Geometry: final body of the model. Coordinates: model frame, mm. A direction names the side the tool comes from. Coordinates: 2 decimals unless noted, no trailing zeros. Order: outer loops, then holes, each group sorted by start corner. A loop starts at its lowest first (then second) coordinate and runs counter-clockwise, first axis right, second up. Notation, with made-up numbers: M 76.5,40 L 104.5,40 A22 cw 104.5,74 Z; hole C 81,16.25 d11. An arc over 180 degrees is marked long. Write item = value, one per line. Start each with the question number.
Autodesk Inventor part; units mm, degrees
ref_plane "YZ Plane" through (0, 0, 0) normal (1, 0, 0) x (0, 1, 0)
ref_plane "XZ Plane" through (0, 0, 0) normal (0, 1, 0) x (-1, 0, 0)
ref_plane "XY Plane" through (0, 0, 0) normal (0, 0, 1) x (1, 0, 0)
sketch "Sketch1" plane through (0, 0, 0) normal (0, 1, 0) x (-1, 0, 0)
  circle A0 centre (0, 0) radius 40
  circle A1 centre (0, 0) radius 36
  dimension "d1" = 72
  dimension "d8" = 80
extrude "Extrusion1" add sketch "Sketch1" along normal blind 50
sketch "Sketch2" plane through (0, 0, 0) normal (1, 0, 0) x (0, 1, 0)
  line L0 (0, 40) -> (0, -40)
  line L1 (0, -36) -> (19.3804, -30.807)
  line L2 (0, -36) -> (20.8201, -41.5787)
  line L3 (19.3804, -30.807) -> (-2.465, -30.807)
  line L4 (-2.465, -30.807) -> (-2.465, -42.37)
  line L5 (-2.465, -42.37) -> (20.8201, -42.37)
  line L6 (20.8201, -42.37) -> (20.8201, -41.5787)
  line L7 (0, -36) -> (50, -36)
  point P0 (0, 0)
  dimension "d6" = 15
  dimension "d7" = 15
extrude "Extrusion2" cut sketch "Sketch2" along normal mid plane 30
properties part number "Whistle Splitter 40mmR"
Item 1: Section query A-A on z = 0. Output: boundary loops of the cut face in (x, y), and give its area (3 significant figures).
Item 2: Section query B-B on x = 3.5. Output: boundary loops of the cut face in (y, z).
Item 3: Section query C-C on y = 7. Output: boundary loops of the cut face in (x, z).
Item 4: Reachability of faces 4 (the flat face through (15, 5, -34)), 5 (the flat face through (-0.21, 5.701, -37.528)), 6 (the flat face through (6, 0, 36)) from +Z, -Z, +X, -X, +Y, -Y: full face, straight path, thin tool, end or side. Return the list, or none.
Item 5: Draft query along X for faces 1 (the flat face through (33, 50, 15)), 2 (the cylindrical face through (4.686, 24.65, -35.694)), 3 (the cylindrical face through (8.67, 24.65, 39.05)). Return one class per face: pulls with the +X half, pulls with the -X half, needs draft (parallel to the pull), parting line crosses it, or undercut.
Item 6: Material intervals for probe 1 along Z at (x, y) = (0, 19); probe 2 along Z at (x, y) = (0, 11.5), sorted ascending. Write a range as [from, to].
Item 7: Section query D-D on x = -16. Output: boundary loops of the cut face in (y, z).
Item 8: First-contact query: pin 1 (12 mm diameter, centred on y = 39, z = 20, fed in from +X); pin 2 (3 mm diameter, centred on x = 22, y = 33, fed in from -Z); pin 3 (2.5 mm diameter, centred on y = 3, z = -35, fed in from -X); pin 4 (6 mm diameter, centred on x = -27.5, z = -15.5, fed in from -Y). Flat tips, straight axial feed; report the tip coordinate or a pass-through.
Ans:
q1.outline = M -40,0 L -36,0 L -36,50 L -40,50 Z; M 36,0 L 40,0 L 40,50 L 36,50 Z
q1.area = 400 mm^2
q2.outline = M 0,-36 L 14.36,-39.85 L 50,-39.85 L 50,-35.83 L 0.64,-35.83 Z; M 0,35.83 L 50,35.83 L 50,39.85 L 0,39.85 Z
q3.outline = M -12.86,-37.88 L 12.86,-37.88 A40 ccw long Z; hole M -15,-34.12 L -11.47,-34.12 A36 ccw 11.47,-34.12 L 15,-34.12 L 15,-32.73 A36 ccw long -15,-32.73 Z
q4.face_4 = -Y
q4.face_5 = -Z, -Y
q4.face_6 = +Z, -Z, +X, -X, -Y
q5.face_1 = needs draft
q5.face_2 = undercut
q5.face_3 = parting line crosses it
q6.probe_1 = [-40, -36], [36, 40]
q6.probe_2 = [-39.08, -36], [36, 40]
q7.outline = M 0,-36.66 L 50,-36.66 L 50,-32.25 L 0,-32.25 Z; M 0,32.25 L 50,32.25 L 50,36.66 L 0,36.66 Z
q8.pin_1 = 37.47
q8.pin_2 = -34.35
q8.pin_3 = -21.47
q8.pin_4 = through
